Work out the finished part from the listing and answer in its coordinate system (mm). Give positions to 0.01 mm unless a question says otherwise; leave off trailing zeros. Order: outer loops, then holes, each group sorted by start corner. A loop starts at its lowest first (then second) coordinate and runs counter-clockwise, first axis right, second up. Notation, with made-up numbers: (52.5, 14) -> (92.5, 14) arc R26 ccw to (92.5, 32) -> close; hole circle Ø2 at (31.5, 3). An arc over 180 degrees is marked (long way). Answer as CSV lines item,"result". Start each with the question number.
1. A cutting plane is placed at A-A (z = 1.15). Give the vertices of the cut face in (x, y).
2. A cutting plane is placed at B-B (y = 3.75). Give the vertices of the cut face in (x, z), then the cut area to 3 significant figures.
3. Find the intervals of material crossed by L1, parallel to X at y = 3.5, z = 1.55; L2, parallel to X at y = 3.25, z = 2.3; L3, parallel to Y at x = 7.25, z = 0.55, in increasing order.
from build123d import *

# Parameters (mm, degrees)
SKETCH_1_W      = 16
SKETCH_1_H      = 7
EXTRUDE_1_DEPTH = 3
CHAMFER_2_SIZE  = 1


with BuildPart() as part:
    # Эскиз1 → Вытянуть1 (new body)
    with BuildSketch(Plane.XY):
        with Locations((0, 0.5)):
            Rectangle(SKETCH_1_W, SKETCH_1_H)
    extrude(amount=EXTRUDE_1_DEPTH)

    # Фаска2
    chamfer_2_edges = [part.edges().sort_by_distance(p)[0] for p in [
        (-8, 4, 1.5),
        (8, 4, 1.5),
        (8, -3, 1.5),
        (-8, -3, 1.5),
    ]]
    chamfer(chamfer_2_edges, length=CHAMFER_2_SIZE)


solid = part.part
Answer sheet:
1,outline,"(-8, -2) -> (-7, -3) -> (7, -3) -> (8, -2) -> (8, 3) -> (7, 4) -> (-7, 4) -> (-8, 3) -> close"
2,outline,"(-7.25, 0) -> (7.25, 0) -> (7.25, 3) -> (-7.25, 3) -> close"
2,area,"43.5 mm^2"
3,L1,"x = -7.5 to 7.5"
3,L2,"x = -7.75 to 7.75"
3,L3,"y = -2.75 to 3.75"
